Autodesk Inventor part; units mm, degrees
ref_plane "YZ Plane" through (0, 0, 0) normal (1, 0, 0) x (0, 1, 0)
ref_plane "XZ Plane" through (0, 0, 0) normal (0, 1, 0) x (-1, 0, 0)
ref_plane "XY Plane" through (0, 0, 0) normal (0, 0, 1) x (1, 0, 0)
sketch "Náčrt1" plane through (0, 0, 0) normal (0, 1, 0) x (-1, 0, 0)
  line L0 (0, 0) -> (116, 0)
  line L1 (116, -40) -> (0, -40)
  circle A0 centre (21, -20) radius 10
  line L2 (116, 0) -> (138, -12.7017)
  line L3 (138, -12.7017) -> (138, -27.2983)
  line L4 (138, -27.2983) -> (116, -40)
  line L5 (0, 0) -> (-5, -5)
  line L6 (-5, -5) -> (-5, -35)
  line L7 (-5, -35) -> (0, -40)
  circle A1 centre (116, -20) radius 8
  circle A2 centre (5, -30) radius 2.5
  circle A3 centre (5, -10) radius 2.5
  dimension "d0" = 5
  dimension "d1" = 5
  dimension "d2" = 5
  dimension "d3" = 143
  dimension "d4" = 16
  dimension "d5" = 20
  dimension "d6" = 40
  dimension "d7" = 20
  dimension "d8" = 26
  dimension "d9" = 30
  dimension "d10" = 95
  dimension "d11" = 121
  dimension "d13" = 30
  dimension "d14" = 20
  dimension "d15" = 5
  dimension "d16" = 5
  dimension "d17" = 10
  dimension "d18" = 10
  dimension "d19" = 10
  dimension "d20" = 10
extrude "Vysunutí1" add sketch "Náčrt1" along normal blind 5
thread "Závit1"
thread "Závit2"
equation "\"d11\" = d10 + d8"
equation "\"d13\" = d9"
properties part number "bočnice"
Geometry: final body of the model. Coordinates: model frame, mm. Coordinates: 2 decimals unless noted, no trailing zeros. Order: outer loops, then holes, each group sorted by start corner. A loop starts at its lowest first (then second) coordinate and runs counter-clockwise, first axis right, second up. Notation, with made-up numbers: (-34.5, 88.25) -> (-9.5, 88.25) arc R33 cw to (-9.5, 124.25) -> close; hole circle Ø11 at (29.5, -11.5). An arc over 180 degrees is marked (long way). Write each question's results on one line, items separated by ' | '. Start each with the question number.
1) Cut plane C-C, the plane x = -5. Output: boundary loops of the cut face in (y, z), and give its area (3 significant figures).
2) Cut plane A-A, the plane y = 2.7. Output: boundary loops of the cut face in (x, z), and give its area (3 significant figures).
3) Cut plane D-D, the plane z = -23. Output: boundary loops of the cut face in (x, y).
4) Cut plane B-B, the plane x = -21. Output: boundary loops of the cut face in (y, z).
5) Mould query, pull axis Z, two halves, no side actions, for faces 1 (the flat face through (-138, 2, -20)), 2 (the cylindrical face through (-30.54, 2.46, -23)), 3 (the flat face through (-126.846, 2.465, -6.262)). Classes: released by +Z, released by -Z, zero draft, split by the parting line, or undercut.
6) Material intervals for line 1 along Z through (x, y) = (-5, 2.15); line 2 along Z through (x, y) = (-21, 1.6); line 3 along X through (y, z) = (1.95, -17.5), sorted ascending.
Checks:
1) outline: (0, -40) -> (5, -40) -> (5, -32.5) -> (0, -32.5) -> close; (0, -27.5) -> (5, -27.5) -> (5, -12.5) -> (0, -12.5) -> close; (0, -7.5) -> (5, -7.5) -> (5, 0) -> (0, 0) -> close | area: 150 mm^2
2) outline: (-138, -27.3) -> (-116, -40) -> (0, -40) -> (5, -35) -> (5, -5) -> (0, 0) -> (-116, 0) -> (-138, -12.7) -> close; hole circle Ø16 at (-116, -20); hole circle Ø20 at (-21, -20); hole circle Ø5 at (-5, -30); hole circle Ø5 at (-5, -10) | area: 4,860 mm^2
3) outline: (-138, 0) -> (-123.42, 0) -> (-123.42, 5) -> (-138, 5) -> close; (-108.58, 0) -> (-30.54, 0) -> (-30.54, 5) -> (-108.58, 5) -> close; (-11.46, 0) -> (5, 0) -> (5, 5) -> (-11.46, 5) -> close
4) outline: (0, -40) -> (5, -40) -> (5, -30) -> (0, -30) -> close; (0, -10) -> (5, -10) -> (5, 0) -> (0, 0) -> close
5) face 1: zero draft | face 2: undercut | face 3: released by +Z
6) line 1: -40 to -32.5, -27.5 to -12.5, -7.5 to 0 | line 2: -40 to -30, -10 to 0 | line 3: -138 to -123.6, -108.4 to -30.68, -11.32 to 5
